Could you check a few things on this drawing? It's one solid part, dimensions in mm from its lowest x, y, z. A direction names the side the tool comes from. Round coordinates to 2 decimals unless told otherwise and drop trailing zeros. Write each loop counter-clockwise with the first axis right and the second up, starting at its lowest first coordinate (ties: lowest second). Pieces come first, ordered by that corner, then holes. Notation, with made-up numbers: M 66,-19.75 L 98,-19.75 A7 ccw 98,-8.75 Z; hole C 22.5,54 d10. An arc over 180 degrees is marked long. One line per item, written item: value. Start each with the question number.
(1) I'm going to push flat-ended pins straight in: pin 1 Ø4 at (y, z) = (6, 13) entering from +X; pin 2 Ø4 at (y, z) = (10, 11) entering from -X; pin 3 Ø6 at (y, z) = (9.5, 14) entering from +X. Where does each tip first touch, or does it pass through?
(2) Which directions (+Z, -Z, +X, -X, +Y, -Y) give clear straight access to the entire face, cutting with the end or side of a thin tool? Please do the marked faces 1 and 2.
(3) If I drill on L1, parallel to Z at x = 2.25, y = 7.25; L2, parallel to Y at x = 5, z = 14; L3, parallel to Y at x = 7.75, z = 1, over which ranges is the centre line in solid material (lowest first)?
(4) I want a section at A-A on z = 18.5. Please give me the cut outline in (x, y), and give its area (3 significant figures).
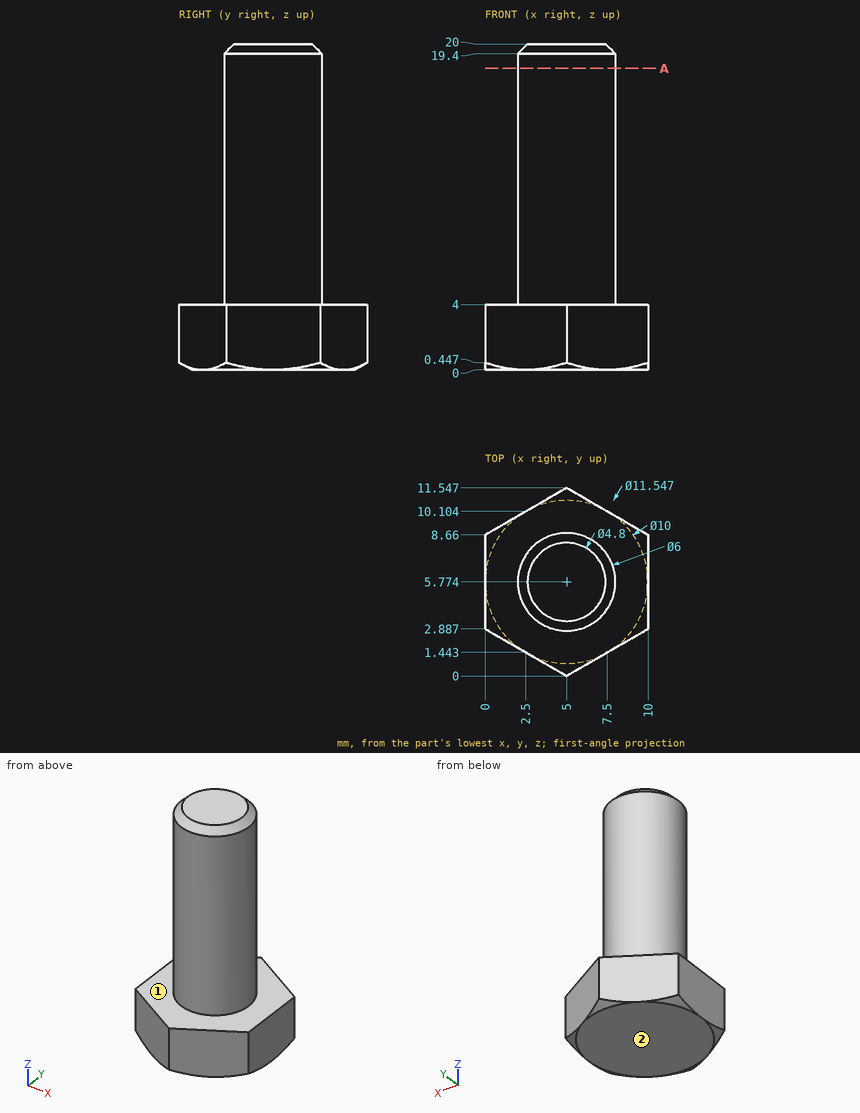
Found:
1. pin 1: stops at x = 8
1. pin 2: stops at x = 2.99
1. pin 3: stops at x = 7.91
2. face 1: +Z
2. face 2: -Z, +X, -X, +Y, -Y
3. L1: z = 0 to 4
3. L2: y = 2.77 to 8.77
3. L3: y = 1.59 to 9.96
4. outline: C 5,5.77 d6
4. area: 28.3 mm²
